from build123d import *

# Parameters (mm, degrees)
SKETCH1_R           = 3.075
BOSS_EXTRUDE1_DEPTH = 5.5
BOSS_EXTRUDE2_START = -6
SKETCH1_3_R         = 6.11
BOSS_EXTRUDE2_DEPTH = 6
BOSS_EXTRUDE3_START = -17
SKETCH1_4_R         = 18.45
BOSS_EXTRUDE3_DEPTH = 11
BOSS_EXTRUDE4_DEPTH = 10
DRAFT1_ANGLE        = 45
BOSS_EXTRUDE5_DEPTH = 3
SKETCH4_R           = 3.075
BOSS_EXTRUDE6_DEPTH = 1.5
SKETCH3_3_R         = 1.55
CUT_EXTRUDE1_DEPTH  = 11
CUT_EXTRUDE2_START  = -7
SKETCH3_4_R         = 1.55
CUT_EXTRUDE2_DEPTH  = 2.6
CUT_EXTRUDE4_START  = -5.5
SKETCH3_5_R         = 1.55
CUT_EXTRUDE4_DEPTH  = 2.5
CUT_EXTRUDE5_START  = -13
CUT_EXTRUDE5_DEPTH  = 13
FILLET1_R           = 3


with BuildPart() as part:
    # Sketch1 → Boss-Extrude1 (new body)
    with BuildSketch(Plane(origin=(57.798756402, 0, 0), x_dir=(0, 0, -1), z_dir=(1, 0, 0))):
        with BuildLine():
            Line((33.998459558, 75.890266162), (78.898459558, 75.890266162))
            Line((78.898459558, 75.890266162), (78.898459558, 120.990266162))
            Line((78.898459558, 120.990266162), (80.735339486, 120.990266162))
            ThreePointArc((80.735339486, 120.990266162), (82.503106439, 121.722499209), (83.235339486, 123.490266162))
            Line((83.235339486, 123.490266162), (83.235339486, 128.990266162))
            Line((83.235339486, 128.990266162), (80.235339486, 128.990266162))
            Line((80.235339486, 128.990266162), (80.235339486, 125.990266162))
            Line((80.235339486, 125.990266162), (15.035339486, 125.990266162))
            Line((15.035339486, 125.990266162), (15.035339486, 128.990266162))
            Line((15.035339486, 128.990266162), (12.035339486, 128.990266162))
            Line((12.035339486, 128.990266162), (12.035339486, 122.990266162))
            ThreePointArc((12.035339486, 122.990266162), (13.49980558, 119.454732256), (17.035339486, 117.990266162))
            Line((17.035339486, 117.990266162), (33.998459558, 117.990266162))
            Line((33.998459558, 117.990266162), (33.998459558, 75.890266162))
        make_face()
        with Locations((49.610967501, 99.839833556)):
            Circle(SKETCH1_R, mode=Mode.SUBTRACT)
    extrude(amount=BOSS_EXTRUDE1_DEPTH)

    # Sketch1<3> → Boss-Extrude2 (add)
    with BuildSketch(Plane(origin=(57.798756402, 0, 0), x_dir=(0, 0, -1), z_dir=(1, 0, 0)).offset(BOSS_EXTRUDE2_START)):
        with BuildLine():
            Line((33.998459558, 75.890266162), (78.898459558, 75.890266162))
            Line((78.898459558, 75.890266162), (78.898459558, 120.990266162))
            Line((78.898459558, 120.990266162), (80.735339486, 120.990266162))
            ThreePointArc((80.735339486, 120.990266162), (82.503106439, 121.722499209), (83.235339486, 123.490266162))
            Line((83.235339486, 123.490266162), (83.235339486, 128.990266162))
            Line((83.235339486, 128.990266162), (80.235339486, 128.990266162))
            Line((80.235339486, 128.990266162), (80.235339486, 125.990266162))
            Line((80.235339486, 125.990266162), (15.035339486, 125.990266162))
            Line((15.035339486, 125.990266162), (15.035339486, 128.990266162))
            Line((15.035339486, 128.990266162), (12.035339486, 128.990266162))
            Line((12.035339486, 128.990266162), (12.035339486, 122.990266162))
            ThreePointArc((12.035339486, 122.990266162), (13.49980558, 119.454732256), (17.035339486, 117.990266162))
            Line((17.035339486, 117.990266162), (33.998459558, 117.990266162))
            Line((33.998459558, 117.990266162), (33.998459558, 75.890266162))
        make_face()
        with Locations(Location((49.610967501, 99.839833556, 0), (0, 0, 90))):
            Circle(SKETCH1_3_R, mode=Mode.SUBTRACT)
    extrude(amount=BOSS_EXTRUDE2_DEPTH)

    # Sketch1<4> → Boss-Extrude3 (add)
    with BuildSketch(Plane(origin=(57.798756402, 0, 0), x_dir=(0, 0, -1), z_dir=(1, 0, 0)).offset(BOSS_EXTRUDE3_START)):
        with BuildLine():
            Line((33.998459558, 75.890266162), (78.898459558, 75.890266162))
            Line((78.898459558, 75.890266162), (78.898459558, 120.990266162))
            Line((78.898459558, 120.990266162), (80.735339486, 120.990266162))
            ThreePointArc((80.735339486, 120.990266162), (82.503106439, 121.722499209), (83.235339486, 123.490266162))
            Line((83.235339486, 123.490266162), (83.235339486, 128.990266162))
            Line((83.235339486, 128.990266162), (80.235339486, 128.990266162))
            Line((80.235339486, 128.990266162), (80.235339486, 125.990266162))
            Line((80.235339486, 125.990266162), (15.035339486, 125.990266162))
            Line((15.035339486, 125.990266162), (15.035339486, 128.990266162))
            Line((15.035339486, 128.990266162), (12.035339486, 128.990266162))
            Line((12.035339486, 128.990266162), (12.035339486, 122.990266162))
            ThreePointArc((12.035339486, 122.990266162), (13.49980558, 119.454732256), (17.035339486, 117.990266162))
            Line((17.035339486, 117.990266162), (33.998459558, 117.990266162))
            Line((33.998459558, 117.990266162), (33.998459558, 75.890266162))
        make_face()
        with Locations(Location((56.448459558, 98.340266162, 0), (0, 0, 90))):
            Circle(SKETCH1_4_R, mode=Mode.SUBTRACT)
    extrude(amount=BOSS_EXTRUDE3_DEPTH)

    # Sketch2 → Boss-Extrude4 (add)
    with BuildSketch(Plane(origin=(40.798756402, 0, 0), x_dir=(0, 0, -1), z_dir=(1, 0, 0))):
        with BuildLine():
            ThreePointArc((69.263798804, 125.990266162), (49.135339486, 132.839833556), (29.006880169, 125.990266162))
            Line((29.006880169, 125.990266162), (69.263798804, 125.990266162))
        make_face()
    extrude(amount=BOSS_EXTRUDE4_DEPTH)

    # Draft1
    draft1_faces = [part.faces().sort_by_distance(p)[0] for p in [
        (50.798756402, 128.756028079, -49.135339486),
    ]]
    draft(draft1_faces, Plane(origin=(152.119080652, 125.990266162, 0), x_dir=(1, 0, 0), z_dir=(0, 1, 0)), DRAFT1_ANGLE)

    # Sketch3 → Boss-Extrude5 (add)
    with BuildSketch(Plane(origin=(0, 125.990266162, 0), x_dir=(1, 0, 0), z_dir=(0, 1, 0))):
        with BuildLine():
            Line((63.298756402, 80.235339486), (59.298756401, 80.235339486))
            ThreePointArc((59.298756401, 80.235339486), (61.860006097, 79.336901605), (63.298756402, 77.035339486))
            Line((63.298756402, 77.035339486), (63.298756402, 80.235339486))
        make_face()
    extrude(amount=BOSS_EXTRUDE5_DEPTH)

    # Sketch4 → Boss-Extrude6 (add)
    with BuildSketch(Plane(origin=(63.298756402, 0, 0), x_dir=(0, 0, -1), z_dir=(1, 0, 0))):
        with BuildLine():
            Line((29.763910038, 128.990266162), (12.035339486, 128.990266162))
            Line((12.035339486, 128.990266162), (12.035339486, 122.990266162))
            ThreePointArc((12.035339486, 122.990266162), (13.49980558, 119.454732256), (17.035339486, 117.990266162))
            Line((17.035339486, 117.990266162), (33.998459558, 117.990266162))
            Line((33.998459558, 117.990266162), (33.998459558, 75.890266162))
            Line((33.998459558, 75.890266162), (78.898459558, 75.890266162))
            Line((78.898459558, 75.890266162), (78.898459558, 120.990266162))
            Line((78.898459558, 120.990266162), (80.735339486, 120.990266162))
            ThreePointArc((80.735339486, 120.990266162), (82.503106439, 121.722499209), (83.235339486, 123.490266162))
            Line((83.235339486, 123.490266162), (83.235339486, 128.990266162))
            Line((83.235339486, 128.990266162), (68.506768934, 128.990266162))
            ThreePointArc((68.506768934, 128.990266162), (70.505131495, 127.558635649), (72.398075234, 125.990266162))
            Line((72.398075234, 125.990266162), (25.872603738, 125.990266162))
            ThreePointArc((25.872603738, 125.990266162), (27.765547478, 127.558635649), (29.763910038, 128.990266162))
        make_face()
        with Locations((49.610967501, 99.839833556)):
            Circle(SKETCH4_R, mode=Mode.SUBTRACT)
    extrude(amount=BOSS_EXTRUDE6_DEPTH)

    # Sketch3<3> → Cut-Extrude1 (cut)
    with BuildSketch(Plane(origin=(0, 125.990266162, 0), x_dir=(1, 0, 0), z_dir=(0, 1, 0))):
        with Locations(Location((49.426066799, 75.535339486, 0), (0, 0, 270))):
            Circle(SKETCH3_3_R)
        with Locations(Location((57.007859867, 75.535339486, 0), (0, 0, 270))):
            Circle(SKETCH3_3_R)
        with Locations(Location((50.298756402, 22.24178562, 0), (0, 0, 180))):
            Circle(SKETCH3_3_R)
    extrude(amount=-CUT_EXTRUDE1_DEPTH, mode=Mode.SUBTRACT)

    # Sketch3<4> → Cut-Extrude2 (cut)
    # profile 1 of 4: a face of its own
    with BuildSketch(Plane(origin=(0, 125.990266162, 0), x_dir=(1, 0, 0), z_dir=(0, 1, 0)).offset(CUT_EXTRUDE2_START)):
        Polygon((54.157859867, 77.180787753), (54.157859867, 73.889891219), (57.007859867, 72.244442952), (59.857859867, 73.889891219), (59.857859867, 77.180787753), (57.007859867, 78.826236021), align=None)
        with Locations(Location((57.007859867, 75.535339486, 0), (0, 0, 270))):
            Circle(SKETCH3_4_R, mode=Mode.SUBTRACT)
    # profile 2 of 4: a face of its own
    with BuildSketch(Plane(origin=(0, 125.990266162, 0), x_dir=(1, 0, 0), z_dir=(0, 1, 0)).offset(CUT_EXTRUDE2_START)):
        Polygon((46.576066799, 77.180787753), (46.576066799, 73.889891219), (49.426066799, 72.244442952), (52.276066799, 73.889891219), (52.276066799, 77.180787753), (49.426066799, 78.826236021), align=None)
        with Locations(Location((49.426066799, 75.535339486, 0), (0, 0, 270))):
            Circle(SKETCH3_4_R, mode=Mode.SUBTRACT)
    # profile 3 of 4: a face of its own
    with BuildSketch(Plane(origin=(0, 125.990266162, 0), x_dir=(1, 0, 0), z_dir=(0, 1, 0)).offset(CUT_EXTRUDE2_START)):
        Polygon((59.857859867, 78.898459558), (59.857859867, 77.180787753), (57.007859867, 78.826236021), (54.157859867, 77.180787753), (54.157859867, 78.898459558), align=None)
    # profile 4 of 4: a face of its own
    with BuildSketch(Plane(origin=(0, 125.990266162, 0), x_dir=(1, 0, 0), z_dir=(0, 1, 0)).offset(CUT_EXTRUDE2_START)):
        Polygon((52.276066799, 78.898459558), (52.276066799, 77.180787753), (49.426066799, 78.826236021), (46.576066799, 77.180787753), (46.576066799, 78.898459558), align=None)
    extrude(amount=-CUT_EXTRUDE2_DEPTH, mode=Mode.SUBTRACT)

    # Sketch3<5> → Cut-Extrude4 (cut)
    with BuildSketch(Plane(origin=(0, 125.990266162, 0), x_dir=(1, 0, 0), z_dir=(0, 1, 0)).offset(CUT_EXTRUDE4_START)):
        Polygon((48.653308134, 19.39178562), (51.944204669, 19.39178562), (53.589652936, 22.24178562), (51.944204669, 25.09178562), (48.653308134, 25.09178562), (47.007859867, 22.24178562), align=None)
        with Locations(Location((50.298756402, 22.24178562, 0), (0, 0, 180))):
            Circle(SKETCH3_5_R, mode=Mode.SUBTRACT)
    extrude(amount=-CUT_EXTRUDE4_DEPTH, mode=Mode.SUBTRACT)

    # Sketch6 → Cut-Extrude5 (cut)
    with BuildSketch(Plane.ZY.offset(-51.798756402).offset(CUT_EXTRUDE5_START)):
        with BuildLine():
            ThreePointArc((-47.52627647, 91.08460293), (-58.402028717, 97.911818335), (-51.38169206, 108.663921867))
            ThreePointArc((-51.38169206, 108.663921867), (-67.681482224, 95.876691159), (-47.52627647, 91.08460293))
        make_face()
    extrude(amount=CUT_EXTRUDE5_DEPTH, mode=Mode.SUBTRACT)

    # Fillet1
    fillet1_edges = [part.edges().sort_by_distance(p)[0] for p in [
        (58.298756402, 91.08460293, -47.52627647),
        (58.298756402, 108.663921867, -51.38169206),
    ]]
    fillet(fillet1_edges, radius=FILLET1_R)


solid = part.part
The listing builds one solid part. Answer for the finished solid, in the listing's coordinates (mm). A direction names the side the tool comes from. Round coordinates to 2 decimals unless told otherwise and drop trailing zeros. Write each loop counter-clockwise with the first axis right and the second up, starting at its lowest first coordinate (ties: lowest second). Pieces come first, ordered by that corner, then holes. Notation, with made-up numbers: (41.25, 88.25) - (58.25, 88.25) arc R12 cw to (58.25, 105.25) - close; hole circle Ø9 at (68.5, 75). An arc over 180 degrees is marked (long way). Use one line per item in the form item = value. Start each with the question number.
Item 1: Determine the mould class of faces 1 (the flat face through (50.831, 117.708, -73.056)), 2 (the flat face through (50, 119, -25.092)), 3 (the flat face through (46.576, 118, -76)) for opening direction Z: +Z half, -Z half, draft (parallel to the pull), parting line (faces both ways), or undercut.
Item 2: A cutting plane is placed at A-A (z = -65.5). Write down the section's boundary in (x, y).
Item 3: Find the intervals of material crossed by line 1 (Z direction, x = 59, y = 98); line 2 (Z direction, x = 53, y = 104.5); line 3 (X direction, y = 86, z = -48), in increasing order. Write a range as [from, to].
Item 4: Flat-ended cylindrical pins translate along their axes: pin 1 Ø1.5 at (y, z) = (107.5, -60.5) entering from -X; pin 2 Ø3 at (x, y) = (61, 106.5) entering from +Z; pin 3 Ø1 at (x, y) = (51, 88.5) entering from -Z; pin 4 Ø2 at (x, z) = (58.5, -80) entering from -Y. Find the tip coordinate at first contact, or state that the pin passes through.
Item 5: A cutting plane is placed at B-B (y = 98). Write down the section's boundary in (x, z), plus the area to 3 significant figures.
Item 6: A tool of negligible diameter and unlimited length cuts with its end or side. For faces 4 (the flat face through (63.299, 128, -21)), 5 (the flat face through (50.1, 118.99, -77.1)), 6 (the flat face through (52, 120.49, -23)), 7 (the cylindrical face through (57.076, 115.7, -77.084)), from which of +Z, -Z, +X, -X, +Y, -Y can it reach the whole face along a straight path? Write none if from no direction.
Item 7: A cutting plane is placed at C-C (y = 82). Write down the section's boundary in (x, z).
The answers:
q1.face_1 = -Z half
q1.face_2 = undercut
q1.face_3 = draft
q2.outline = (40.8, 75.89) - (64.8, 75.89) - (64.8, 91.25) - (51.8, 91.25) - (51.8, 82.26) - (40.8, 82.26) - close; (40.8, 114.42) - (51.8, 114.42) - (51.8, 105.43) - (64.8, 105.43) - (64.8, 125.99) - (50.8, 125.99) - (48.29, 128.5) - (40.8, 128.5) - close
q3.line_1 = [-78.9, -67.94], [-58.42, -52.07], [-47.15, -34]
q3.line_2 = [-78.9, -66.16], [-57.31, -53.56], [-45.66, -34]
q3.line_3 = [51.8, 64.8]
q4.pin_1 = through
q4.pin_2 = -34
q4.pin_3 = -78.9
q4.pin_4 = 120.99
q5.outline = (40.8, -78.9) - (64.8, -78.9) - (64.8, -67.94) - (51.8, -67.94) - (51.8, -74.9) - (40.8, -74.9) - close; (40.8, -38) - (51.8, -38) - (51.8, -43.78) - (57.8, -43.78) - (57.8, -47.15) - (64.8, -47.15) - (64.8, -34) - (40.8, -34) - close; (51.8, -58.42) - (64.8, -58.42) - (64.8, -52.07) - (57.8, -52.07) - (57.8, -55.44) - (51.8, -55.44) - close
q5.area = 444 mm^2
q6.face_4 = -X, +Y
q6.face_5 = -Z
q6.face_6 = -Y
q6.face_7 = +Y
q7.outline = (40.8, -78.9) - (64.8, -78.9) - (64.8, -34) - (40.8, -34) - (40.8, -47.88) - (51.8, -47.88) - (51.8, -65.02) - (40.8, -65.02) - close
